Can you work these out from the model? Positions are in its coordinate system, mm. A direction names the side the tool comes from. Give positions to 0.01 mm unless a question says otherwise; leave off trailing zeros. Write each loop counter-clockwise with the first axis right and the second up, starting at its lowest first coordinate (ties: lowest second). Pieces come first, ordered by that corner, then holes. Notation, with made-up numbers: (-4, 15) -> (11, 15) arc R22 cw to (11, 39) -> close; hole circle Ø4 at (14, 65.5). An arc over 180 degrees is marked (long way). Answer as CSV lines item,"result". Start each with the question number.
1. If we mould it in two halves opening along Z, with no side actions, what happens to faces 1 (the face through (0, -8, -8)), 2 (the face through (-6.07, 35.694, -4.686)), 3 (the face through (-8.89, 9.76, -2.17))? For each: pulls with the +Z half, pulls with the -Z half, needs draft (parallel to the pull), parting line crosses it, or undercut.
2. I'm going to push flat-ended pins straight in: P1, Ø10.5, axis at y = 0, z = 28, coming from the +X side; P2, Ø1, axis at x = -11.5, z = 4, coming from the +Y side; P3, Ø6, axis at x = -10.5, z = 12.5, coming from the -Y side; P4, Ø6, axis at x = -10, z = 18.5, coming from the +Y side. Where does each tip first touch, or does it pass through?
3. If we section it at A-A on z = 0: Count the separate pieces of the cut face and the enclosed holes in it, plus the area to 3 significant figures.
4. On a 3-axis mill with a long thin cutter (end or side, diameter ignored), from which of +Z, -Z, +X, -X, +Y, -Y can I reach the whole of each face in a straight line? I mean faces 4 (the face through (-5.9, -2.4, 31.2)), 5 (the face through (-12, 15, 15)). Say none if no direction works.
5. I need wall thicknesses on line 1 (Y direction, x = -6, z = 0); line 2 (X direction, y = 20, z = 15.5); line 3 (Y direction, x = -5.75, z = 27). Which ranges of each line are inside material? Lowest first, please. Write a range as [from, to].
6. If we section it at B-B on x = -6.5: Write out the boundary of the cut face in (y, z).
Solid Edge part; units mm, degrees
sketch "Sketch1" plane through (0, 0, 0) normal (0, -1, 0) x (1, 0, 0)
  line L0 (0, 10) -> (0, 36)
  line L1 (0, 36) -> (-12, 36)
  line L2 (-12, 20) -> (-12, 36)
  line L3 (-18, 20) -> (-12, 20)
  line L4 (-18, 10) -> (-18, 20)
  line L5 (-18, 10) -> (0, 10)
revolve "RevolvedProtrusion1" add sketch "Sketch1" angle 360 about axis through (-60, 0, 0) along (1, 0, 0)
sketch "Sketch2" plane through (0, 0, 0) normal (1, 0, 0) x (0, 0, -1)
  circle A0 centre (0, 28) radius 4
  circle A1 centre (-28, 0) radius 4
  circle A2 centre (0, -28) radius 4
  circle A3 centre (28, 0) radius 4
extrude "Cutout1" cut sketch "Sketch2" against normal blind 30
fillet "Round_1" radius 1 5 edges at (0, 0, -36) (-12, 0, -36) (-18, 0, -20) (-18, 0, -10) (0, 0, -10)
Computed values:
1,face 1,"needs draft"
1,face 2,"parting line crosses it"
1,face 3,"undercut"
2,P1,"stops at x = 0"
2,P2,"stops at y = 35.8"
2,P3,"stops at y = -34.72"
2,P4,"stops at y = 32.49"
3,separate pieces,"4"
3,enclosed holes,"0"
3,area,"550 mm2"
4,face 4,"+X, -X"
4,face 5,"-X"
5,line 1,"y = [-36, -32], [-24, -10], [10, 24], [32, 36]"
5,line 2,"x = [-12, 0]"
5,line 3,"y = [-23.81, -3.87], [3.87, 23.81]"
6,outline,"circle Ø72 at (0, 0); hole circle Ø8 at (-28, 0); hole circle Ø20 at (0, 0); hole circle Ø8 at (0, -28); hole circle Ø8 at (0, 28); hole circle Ø8 at (28, 0)"
